```python
from build123d import *

# Parameters (mm, degrees)
SKETCH1_W                      = 203.2
SKETCH1_H                      = 60
SKETCH1_R                      = 3.3
SKETCH1_R_2                    = 3.5
BOSS_EXTRUDE1_DEPTH            = 3.175
SKETCH2_R                      = 3.2639
F_1_4_20_FOR_NUT_BRACKET_DEPTH = 106.984152707
SKETCH3_R                      = 0.79375
SKETCH3_R_2                    = 3.2639
WIRE_HOLDER_DEPTH              = 106.984152707


with BuildPart() as part:
    # Sketch1 → Boss-Extrude1 (new body)
    with BuildSketch(Plane(origin=(0, 0, 0), x_dir=(1, 0, 0), z_dir=(0, 1, 0))):
        Rectangle(SKETCH1_W, SKETCH1_H)
        with Locations(Location((-52.4, 20, 0), (0, 0, 270))):
            Circle(SKETCH1_R, mode=Mode.SUBTRACT)
        with Locations(Location((-92.4, -20, 0), (0, 0, 90))):
            Circle(SKETCH1_R_2, mode=Mode.SUBTRACT)
        with Locations(Location((-52.4, -20, 0), (0, 0, 90))):
            Circle(SKETCH1_R, mode=Mode.SUBTRACT)
        with Locations(Location((92.4, 20, 0), (0, 0, 90))):
            Circle(SKETCH1_R_2, mode=Mode.SUBTRACT)
        with Locations(Location((-92.4, 20, 0), (0, 0, 270))):
            Circle(SKETCH1_R_2, mode=Mode.SUBTRACT)
        with Locations(Location((52.4, -20, 0), (0, 0, 270))):
            Circle(SKETCH1_R, mode=Mode.SUBTRACT)
        with Locations(Location((92.4, -20, 0), (0, 0, 270))):
            Circle(SKETCH1_R_2, mode=Mode.SUBTRACT)
        with Locations(Location((52.4, 20, 0), (0, 0, 90))):
            Circle(SKETCH1_R, mode=Mode.SUBTRACT)
    extrude(amount=BOSS_EXTRUDE1_DEPTH)

    # Sketch2 → 1/4-20 for Nut Bracket (cut, through all)
    with BuildSketch(Plane(origin=(0, 3.175, 0), x_dir=(1, 0, 0), z_dir=(0, 1, 0))):
        with Locations(Location((-12.7, -17.3, 0), (0, 0, 270))):
            Circle(SKETCH2_R)
        with Locations(Location((12.7, -17.3, 0), (0, 0, 270))):
            Circle(SKETCH2_R)
        with Locations(Location((0, 0.48, 0), (0, 0, 270))):
            Circle(SKETCH2_R)
    extrude(amount=-F_1_4_20_FOR_NUT_BRACKET_DEPTH, mode=Mode.SUBTRACT)

    # Sketch3 → Wire Holder (cut, through all)
    with BuildSketch(Plane(origin=(0, 3.175, 0), x_dir=(1, 0, 0), z_dir=(0, 1, 0))):
        with Locations(Location((31.6, -15, 0), (0, 0, 270))):
            Circle(SKETCH3_R)
        with Locations(Location((36.6, 15, 0), (0, 0, 270))):
            Circle(SKETCH3_R_2)
    extrude(amount=-WIRE_HOLDER_DEPTH, mode=Mode.SUBTRACT)


solid = part.part
```
CAD build for the part. Positions are in the model's coordinates, mm. Give positions to 0.01 mm unless a question says otherwise; leave off trailing zeros. Write each loop counter-clockwise with the first axis right and the second up, starting at its lowest first coordinate (ties: lowest second). Pieces come first, ordered by that corner, then holes. Notation, with made-up numbers: M 87,3 L 124,3 A22 cw 124,29 Z; hole C -14.5,28.25 d7. An arc over 180 degrees is marked long. Return JSON: item names as keys, results as strings. Group by question number.
(1) Mould opens along X. For faces 1 (the face through (-55.62, 1.57, -20.72)), 2 (the face through (-1, 3.175, -7)) say: pulls with the +X half, pulls with the -X half, needs draft (parallel to the pull), parting line crosses it, or undercut.
(2) Drill centre lines: L1, parallel to X at y = 1.65, z = -15; L2, parallel to Z at x = 14, y = 2.1; L3, parallel to Z at x = 89.5, y = 0.75. Where is each one in solid material? Low to high. Write a range as [from, to].
(3) Band-saw the part on B-B (x = 0). Give the cut face in (y, z) (3 decimals), and give its area (3 significant figures).
(4) Band-saw the part on A-A (x = -92.4). Give the cut face in (y, z) (3 decimals).
(5) Band-saw the part on C-C (z = -20). Give the cut face in (x, y) (3 decimals).
(6) Band-saw the part on D-D (y = 0.6). State how many separate pieces and enclosed holes the cut face has, and give its area (3 significant figures).
Entries:
{
 "1": {"face 1": "undercut", "face 2": "needs draft"},
 "2": {"L1": "x = [-101.6, 33.34], [39.86, 101.6]", "L2": "z = [-30, 14.31], [20.29, 30]", "L3": "z = [-30, -21.96], [-18.04, 18.04], [21.96, 30]"},
 "3": {"outline": "M 0,-30 L 3.175,-30 L 3.175,-3.744 L 0,-3.744 Z; M 0,2.784 L 3.175,2.784 L 3.175,30 L 0,30 Z", "area": "170 mm^2"},
 "4": {"outline": "M 0,-30 L 3.175,-30 L 3.175,-23.5 L 0,-23.5 Z; M 0,-16.5 L 3.175,-16.5 L 3.175,16.5 L 0,16.5 Z; M 0,23.5 L 3.175,23.5 L 3.175,30 L 0,30 Z"},
 "5": {"outline": "M -101.6,0 L -95.9,0 L -95.9,3.175 L -101.6,3.175 Z; M -88.9,0 L -55.7,0 L -55.7,3.175 L -88.9,3.175 Z; M -49.1,0 L 49.1,0 L 49.1,3.175 L -49.1,3.175 Z; M 55.7,0 L 88.9,0 L 88.9,3.175 L 55.7,3.175 Z; M 95.9,0 L 101.6,0 L 101.6,3.175 L 95.9,3.175 Z"},
 "6": {"separate pieces": "1", "enclosed holes": "13", "area": "11,800 mm^2"}
}
